Design review of the part shown in the three views and the two pictorial views. Dimensions are in mm from the part's minimum x, y and z. A direction names the side the tool comes from. Coordinates: 2 decimals unless noted, no trailing zeros. Loops run counter-clockwise (first coordinate to the right, second up) from the corner with the lowest first, then second, coordinate; pieces in that order, holes last. Notation, with made-up numbers: M 75,78 L 80,78 A36 ccw 80,116 Z; hole C 83.5,-17.75 d4. An arc over 180 degrees is marked long. Use one line per item in the form item = value.
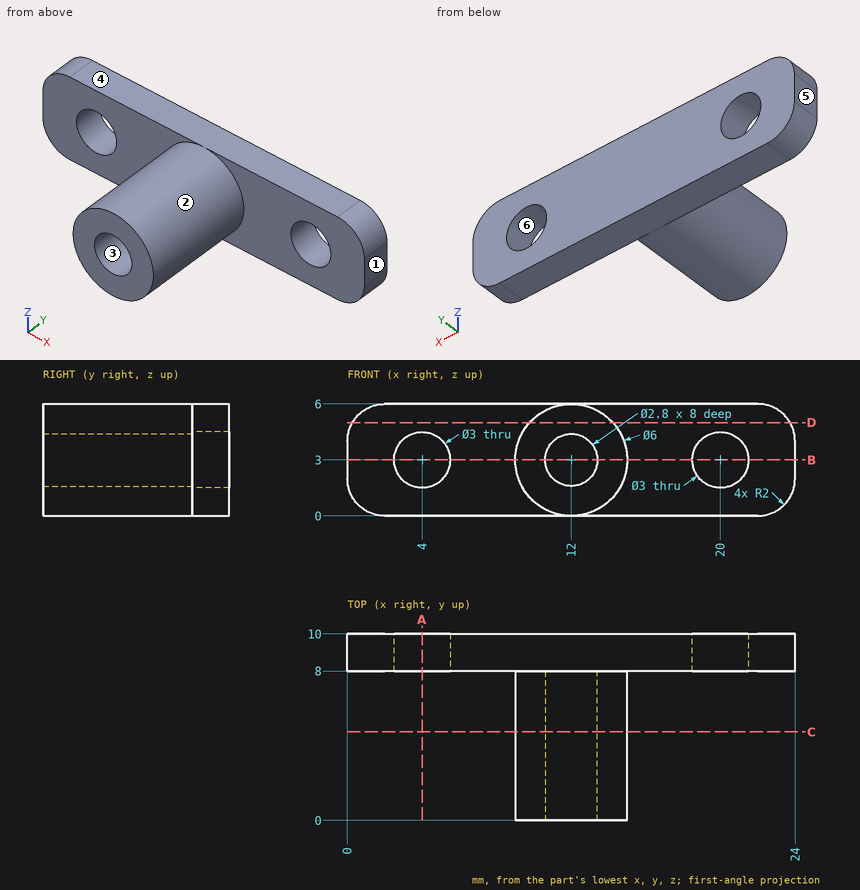
1. Add section B-B (z = 3). State the section outline as (x, y) points.
Response values:
outline = M 0,8 L 2.5,8 L 2.5,10 L 0,10 Z; M 5.5,8 L 9,8 L 9,0 L 10.6,0 L 10.6,8 L 13.4,8 L 13.4,0 L 15,0 L 15,8 L 18.5,8 L 18.5,10 L 5.5,10 Z; M 21.5,8 L 24,8 L 24,10 L 21.5,10 Z
2. Wall thickness on line 1 along Z through (x, y) = (12, 3.75); line 2 along Z through (x, y) = (20, 8.75); line 3 along X through (y, z) = (8.5, 3.9): over which ranges is each line inside the solid? List them lowest first. Write a range as from..to.
Response values:
line_1 = 0..1.6, 4.4..6
line_2 = 0..1.5, 4.5..6
line_3 = 0..2.8, 5.2..18.8, 21.2..24
3. Add section A-A (x = 4). State the section outline as (y, z) points.
Response values:
outline = M 8,0 L 10,0 L 10,1.5 L 8,1.5 Z; M 8,4.5 L 10,4.5 L 10,6 L 8,6 Z
4. The part is to be moulded in two halves that separate along X. For the marked faces 3, 4, 5 and 6, say which applies: pulls with the +X half, pulls with the -X half, needs draft (parallel to the pull), parting line crosses it, or undercut.
Response values:
face_3 = undercut
face_4 = needs draft
face_5 = pulls with the -X half
face_6 = undercut
5. Add section C-C (y = 4.75). State the section outline as (x, z) points, then the cut area to 3 significant figures.
Response values:
outline = C 12,3 d6; hole C 12,3 d2.8
area = 22.1 mm^2
6. Insertion check: P1, Ø1.7, axis at x = 12, z = 3, coming from the -Y side; P2, Ø3, axis at y = 3, z = 4, coming from the -X side. Each pin has a flat end and moves straight along its axis. Give the tip position at first contact, or say it passes through.
Response values:
P1 = 8
P2 = 9
7. Machinability: for the marked faces 1 and 2, which of the approach directions +Z, -Z, +X, -X, +Y, -Y give a long, thin tool a straight path to every point of the face, cutting with its end or side? Answer none if there is none.
Response values:
face_1 = +Z, -Z, +X, +Y, -Y
face_2 = -Y
8. Add section D-D (z = 5). State the section outline as (x, y) points, then the cut area to 3 significant figures.
Response values:
outline = M 0.27,8 L 9.76,8 L 9.76,0 L 14.24,0 L 14.24,8 L 23.73,8 L 23.73,10 L 0.27,10 Z
area = 82.7 mm^2
